Check sheet for the modelled part. Datum: model origin and axes. Units: mm. A direction names the side the tool comes from. Round coordinates to 2 decimals unless told otherwise and drop trailing zeros. Loops run counter-clockwise (first coordinate to the right, second up) from the corner with the lowest first, then second, coordinate; pieces in that order, holes last. Notation, with made-up numbers: M 86,0 L 110,0 A29 ccw 110,34 Z; hole C -26.5,14 d11. An arc over 180 degrees is marked long. One line per question, with ' | ' between items. Start each with the question number.
(1) Draft check along Z on faces 6 (the face through (-72.094, -82.283, -14.402)), 7 (the face through (76, -101.6, -13)), 8 (the face through (-55.125, -114.122, -18.669)), 9 (the face through (80.306, -82.817, -14.402)). Enter one of: +Z half, -Z half, draft (parallel to the pull), parting line (faces both ways), or undercut.
(2) Section check B-B (y = -94). Record the boundary of the cut face in (x, z) (3 decimals).
(3) Go/stop test with flat-tipped pins: P1, Ø12.5, axis at x = 46.5, z = -15, coming from the -Y side; P2, Ø2.5, axis at x = 77, z = -12.5, coming from the -Y side; P3, Ø3, axis at x = -27, y = 71, coming from the -Z side. Record where each tip stops, or that it passes through.
(4) Thickness scan on probe 1 along Y at (x, z) = (-91, -21); probe 2 along Z at (x, y) = (-25.5, -7.5); probe 3 along Z at (x, y) = (-126, -9). Record the ranges inside material, lowest first. Write a range as [from, to].
(5) Section check A-A (x = -8.5). Record the boundary of the cut face in (y, z).
(6) Tool access check on faces 1 (the face through (-76, -127, -50)), 2 (the face through (101.6, 1, -13)), 3 (the face through (-76, 101.6, -13)), 4 (the face through (-1, -1, -25.4)), 5 (the face through (-72.094, 82.283, -14.402)). Record the directions out of +Z, -Z, +X, -X, +Y, -Y that give a thin tool (end or side, any length) a straight path to the whole face; none if there is none.
(7) Section check D-D (z = -59). Record the boundary of the cut face in (x, y), and give its area (3 significant figures).
(8) Section check C-C (y = -44). Record the boundary of the cut face in (x, z), and give its area (3 significant figures).
```python
from build123d import *

# Parameters (mm, degrees)
F0_W     = 304.8
F0_H     = 203.2
F1_DEPTH = 3
F2_W     = 203.2
F2_H     = 127
F3_DEPTH = 25.4
F4_R     = 4.445
F5_DEPTH = 101.6
F6_R     = 38.1
F7_DEPTH = 25.4


with BuildPart() as f1:
    # F0 (on Top) → F1 (new body)
    with BuildSketch(Plane.XY):
        Rectangle(F0_W, F0_H)
    extrude(amount=F1_DEPTH)

    # F2 (on face) → F3 (join)
    with BuildSketch(Plane(origin=(0, 0, 0), x_dir=(1, 0, 0), z_dir=(0, 0, -1))):
        Rectangle(F2_W, F2_H)
    extrude(amount=F3_DEPTH)

    # F4 (on Front) → F5 (join, symmetric)
    with BuildSketch(Plane.XZ):
        with Locations((-76.2, -12.7)):
            Circle(F4_R)
        with Locations((76.2, -12.7)):
            Circle(F4_R)
    extrude(amount=F5_DEPTH, both=True)

    # F6 (on face) → F7 (join)
    with BuildSketch(Plane.XZ.offset(101.6)):
        with Locations((-75.607116, -50.795387)):
            Circle(F6_R)
    extrude(amount=F7_DEPTH)


solid = f1.part
```
The answers:
1) face 6: undercut | face 7: draft | face 8: parting line | face 9: undercut
2) outline: M -152.4,0 L 152.4,0 L 152.4,3 L -152.4,3 Z; C -76.2,-12.7 d8.89; C 76.2,-12.7 d8.89
3) P1: y = -63.5 | P2: y = -101.6 | P3: z = 0
4) probe 1: [-127, -101.6], [-63.5, 63.5] | probe 2: [-25.4, 3] | probe 3: [0, 3]
5) outline: M -101.6,0 L -63.5,0 L -63.5,-25.4 L 63.5,-25.4 L 63.5,0 L 101.6,0 L 101.6,3 L -101.6,3 Z
6) face 1: +Z, -Z, +X, -X, -Y | face 2: -Z, +X, +Y, -Y | face 3: +Z, -Z, +X, -X, +Y | face 4: -Z, +X, -X, +Y | face 5: +Y
7) outline: M -112.81,-127 L -38.4,-127 L -38.4,-101.6 L -112.81,-101.6 Z | area: 1,890 mm²
8) outline: M -152.4,0 L -101.6,0 L -101.6,-25.4 L 101.6,-25.4 L 101.6,0 L 152.4,0 L 152.4,3 L -152.4,3 Z | area: 6,080 mm²
